For this review, take the finished solid that the model builds, in its own axes (mm). A direction names the side the tool comes from. Round coordinates to 2 decimals unless told otherwise and drop trailing zeros. Write each loop counter-clockwise with the first axis right and the second up, starting at its lowest first coordinate (ties: lowest second). Pieces come first, ordered by that corner, then holes. Notation, with made-up numbers: M 82.5,71 L 86.5,71 A11 ccw 86.5,80 Z; hole C 12,-20 d8. An arc over 180 degrees is marked long. One line per question, with ' | ' between items.
```python
from build123d import *

# Parameters (mm, degrees)
SALIENTE_EXTRUIR1_DEPTH    = 2.125
CROQUIS3_R                 = 2
CORTAR_EXTRUIR1_DEPTH      = 1
CORTAR_EXTRUIR1_DEPTH_BACK = 10
CHAMFER1_SIZE              = 2.1


with BuildPart() as part:
    # Croquis1 → Saliente-Extruir1 (new body, symmetric)
    with BuildSketch(Plane.XY):
        Polygon((0, 0), (100, 0), (129.7, 30), (69.7, 30), align=None)
    extrude(amount=SALIENTE_EXTRUIR1_DEPTH, both=True)

    # Croquis3 → Cortar-Extruir1 (cut, two sides)
    with BuildSketch(Plane.XZ) as cortar_extruir1_sk:
        with Locations((73, 0)):
            Circle(CROQUIS3_R)
    extrude(amount=CORTAR_EXTRUIR1_DEPTH, mode=Mode.SUBTRACT)
    extrude(cortar_extruir1_sk.sketch, amount=-CORTAR_EXTRUIR1_DEPTH_BACK, mode=Mode.SUBTRACT)

    # Chamfer1
    chamfer1_edges = [part.edges().sort_by_distance(p)[0] for p in [
        (114.85, 15, 2.125),
        (99.7, 30, 2.125),
        (34.85, 15, 2.125),
        (99.7, 30, -2.125),
        (114.85, 15, -2.125),
        (34.85, 15, -2.125),
    ]]
    chamfer(chamfer1_edges, length=CHAMFER1_SIZE)


solid = part.part
```
Item 1: Take a section at D-D (x = 37.5). Write out the cut boundary in (y, z) (3 decimals).
Results:
outline: M 0,-2.125 L 13.854,-2.125 L 16.141,-0.025 L 16.141,0.025 L 13.854,2.125 L 0,2.125 Z
Item 2: To check wall thickness, follow line 1 along Y through (x, z) = (102, 0.15) (3 decimals); line 2 along Y through (x, z) = (40.5, 1.5); line 3 along Z through (x, y) = (109, 29.5) (3 decimals). State the ranges of each line that lie inside material, in increasing order. Write a range as from..to.
Results:
line 1: 2.198..29.875 | line 2: 0..15.83 | line 3: -0.525..0.525
Item 3: Mouldability with a two-part tool opening along X and no side actions: class faces 3 (the face through (73, 10, 0)), 4 (the face through (113.165, 14.769, -1.06)), 5 (the face through (35.76, 14.23, 1.09)), 6 (the face through (77, 14, 2.125)) as +X half, -X half, draft (parallel to the pull), parting line (faces both ways), or undercut.
Results:
face 3: undercut | face 4: +X half | face 5: -X half | face 6: draft
Item 4: Take a section at C-C (z = -0.9). Write out the cut boundary in (x, y) (3 decimals), then the cut area to 3 significant figures.
Results:
outline: M 2.213,0 L 71.214,0 L 71.214,10 L 74.786,10 L 74.786,0 L 98.769,0 L 127.602,29.125 L 69.88,29.125 Z | area: 2,210 mm2
Item 5: Insertion check: pin 1 Ø2 at (x, z) = (73.5, 0.5) entering from -Y. The pin has a flat end and moves straight along its axis. Give the tip position at first contact, or say it passes through.
Results:
pin 1: y = 10
Item 6: Take a section at B-B (y = 25.5). Write out the cut boundary in (x, z) (3 decimals).
Results:
outline: M 59.245,-0.025 L 64.557,-2.125 L 122.29,-2.125 L 125.245,-0.025 L 125.245,0.025 L 122.29,2.125 L 64.557,2.125 L 59.245,0.025 Z
Item 7: Take a section at A-A (x = 73). Write out the cut boundary in (y, z) (3 decimals).
Results:
outline: M 0,-2.125 L 27.9,-2.125 L 30,-0.025 L 30,0.025 L 27.9,2.125 L 0,2.125 L 0,2 L 10,2 L 10,-2 L 0,-2 Z
Item 8: Machinability: for faces 1 (the face through (49, 0, 0)), 2 (the face through (74.908, 4.93, 0.601)), which of the approach directions +Z, -Z, +X, -X, +Y, -Y give a long, thin tool a straight path to every point of the face, cutting with its end or side? Answer none if there is none.
Results:
face 1: +Z, -Z, +X, -X, -Y | face 2: -Y
